```python
from build123d import *

# Parameters (mm, degrees)
ESQUISSE1_R             = 150
BOSS_EXTRU_1_DEPTH      = 2
ESQUISSE1_4_R           = 1.25
ENL_V_MAT_EXTRU_1_DEPTH = 1
ESQUISSE1_5_R           = 1.25
ENL_V_MAT_EXTRU_2_DEPTH = 13
BOSS_EXTRU_3_START      = 3
BOSS_EXTRU_3_DEPTH      = 3
BOSS_EXTRU_4_DEPTH      = 3
ENL_V_MAT_EXTRU_3_DEPTH = 50
CONG_1_R                = 1
ESQUISSE5_R             = 1
ENL_V_MAT_EXTRU_4_DEPTH = 180
ENL_V_MAT_EXTRU_5_DEPTH = 213.153246642
ESQUISSE7_W             = 7
ESQUISSE7_H             = 1
BOSS_EXTRU_5_DEPTH      = 20
CONG_3_R                = 1


with BuildPart() as part:
    # Esquisse1 → Boss.-Extru.1 (new body)
    with BuildSketch(Plane(origin=(0, 0, 0), x_dir=(1, 0, 0), z_dir=(0, 1, 0))):
        with Locations(Location((0, 0, 0), (0, 0, 270))):
            Circle(ESQUISSE1_R)
    extrude(amount=-BOSS_EXTRU_1_DEPTH)

    # Esquisse1<4> → Enlèv. mat.-Extru.1 (cut)
    with BuildSketch(Plane(origin=(0, 0, 0), x_dir=(1, 0, 0), z_dir=(0, 1, 0))):
        with BuildLine():
            Line((120, -88.323269867), (120, 88.323269867))
            ThreePointArc((120, 88.323269867), (-149, 0), (120, -88.323269867))
        make_face()
        with Locations(Location((0, -18.4, 0), (0, 0, 270))):
            Circle(ESQUISSE1_4_R, mode=Mode.SUBTRACT)
        with Locations(Location((0, -11, 0), (0, 0, 270))):
            Circle(ESQUISSE1_4_R, mode=Mode.SUBTRACT)
        Polygon((5, 7), (5, -6.999999465), (-5, -7), (-5.000000382, 7), align=None, mode=Mode.SUBTRACT)
        with Locations(Location((0, 11, 0), (0, 0, 270))):
            Circle(ESQUISSE1_4_R, mode=Mode.SUBTRACT)
        with Locations(Location((0, 18.4, 0), (0, 0, 270))):
            Circle(ESQUISSE1_4_R, mode=Mode.SUBTRACT)
    extrude(amount=-ENL_V_MAT_EXTRU_1_DEPTH, mode=Mode.SUBTRACT)

    # Esquisse1<5> → Enlèv. mat.-Extru.2 (cut)
    with BuildSketch(Plane(origin=(0, 0, 0), x_dir=(1, 0, 0), z_dir=(0, 1, 0))):
        Polygon((5, -6.999999465), (5, 7), (-5.000000382, 7), (-5, -7), align=None)
        with Locations(Location((0, -11, 0), (0, 0, 270))):
            Circle(ESQUISSE1_5_R)
        with Locations(Location((0, -18.4, 0), (0, 0, 270))):
            Circle(ESQUISSE1_5_R)
        with Locations(Location((0, 11, 0), (0, 0, 270))):
            Circle(ESQUISSE1_5_R)
        with Locations(Location((0, 18.4, 0), (0, 0, 270))):
            Circle(ESQUISSE1_5_R)
    extrude(amount=-ENL_V_MAT_EXTRU_2_DEPTH, mode=Mode.SUBTRACT)

    # Esquisse3 → Boss.-Extru.3 (add)
    with BuildSketch(Plane(origin=(0, 0, 0), x_dir=(1, 0, 0), z_dir=(0, 1, 0)).offset(BOSS_EXTRU_3_START)):
        with BuildLine():
            Line((120, -3.5), (149.959161107, -3.5))
            ThreePointArc((149.959161107, -3.5), (149.989789929, -1.750119126), (150, 0))
            ThreePointArc((150, 0), (149.989789929, 1.750119126), (149.959161107, 3.5))
            Line((149.959161107, 3.5), (120, 3.5))
            Line((120, 3.5), (120, -3.5))
        make_face()
    extrude(amount=-BOSS_EXTRU_3_DEPTH)

    # Esquisse3<2> → Boss.-Extru.4 (add)
    with BuildSketch(Plane(origin=(0, 0, 0), x_dir=(1, 0, 0), z_dir=(0, 1, 0))):
        with BuildLine():
            Line((120, -3.5), (149.959161107, -3.5))
            ThreePointArc((149.959161107, -3.5), (149.989789929, -1.750119126), (150, 0))
            ThreePointArc((150, 0), (149.989789929, 1.750119126), (149.959161107, 3.5))
            Line((149.959161107, 3.5), (120, 3.5))
            Line((120, 3.5), (120, -3.5))
        make_face()
    extrude(amount=-BOSS_EXTRU_4_DEPTH)

    # Esquisse4 → Enlèv. mat.-Extru.3 (cut)
    with BuildSketch(Plane(origin=(120, 0, 0), x_dir=(0, 0, -1), z_dir=(1, 0, 0))):
        with BuildLine():
            Line((-2, 1.5), (2, 1.5))
            ThreePointArc((2, 1.5), (2.5, 0), (2, -1.5))
            Line((2, -1.5), (-2, -1.5))
            ThreePointArc((-2, -1.5), (-2.5, 0), (-2, 1.5))
        make_face()
    extrude(amount=ENL_V_MAT_EXTRU_3_DEPTH, mode=Mode.SUBTRACT)

    # Congé1
    cong_1_edges = [part.edges().sort_by_distance(p)[0] for p in [
        (134.979580554, -3, -3.5),
        (134.979580554, -3, 3.5),
        (134.979580554, 3, 3.5),
        (134.979580554, 3, -3.5),
    ]]
    fillet(cong_1_edges, radius=CONG_1_R - 0.0001)  # a hair under: the kernel refuses the full size

    # Esquisse5 → Enlèv. mat.-Extru.4 (cut)
    with BuildSketch(Plane(origin=(0, 0, 0), x_dir=(0, 0, -1), z_dir=(1, 0, 0))):
        Circle(ESQUISSE5_R)
    extrude(amount=-ENL_V_MAT_EXTRU_4_DEPTH, mode=Mode.SUBTRACT)

    # Esquisse3<4> → Enlèv. mat.-Extru.5 (cut, through all)
    with BuildSketch(Plane(origin=(0, 0, 0), x_dir=(1, 0, 0), z_dir=(0, 1, 0))):
        with BuildLine():
            ThreePointArc((149.959161107, 3.5), (-150, 0), (149.959161107, -3.5))
            Line((149.959161107, -3.5), (120, -3.5))
            Line((120, -3.5), (120, -88.323269867))
            ThreePointArc((120, -88.323269867), (-149, 0), (120, 88.323269867))
            Line((120, 88.323269867), (120, 3.5))
            Line((120, 3.5), (149.959161107, 3.5))
        make_face()
    extrude(amount=-ENL_V_MAT_EXTRU_5_DEPTH, mode=Mode.SUBTRACT)

    # Esquisse7 → Boss.-Extru.5 (add)
    with BuildSketch(Plane.ZY.offset(-120)):
        with Locations((0, -2.5)):
            Rectangle(ESQUISSE7_W, ESQUISSE7_H)
    extrude(amount=BOSS_EXTRU_5_DEPTH)

    # Congé3
    cong_3_edges = [part.edges().sort_by_distance(p)[0] for p in [
        (100, -3, 0),
        (110, -3, -3.5),
        (110, -3, 3.5),
    ]]
    fillet(cong_3_edges, radius=CONG_3_R - 0.0001)  # a hair under: the kernel refuses the full size


solid = part.part
```
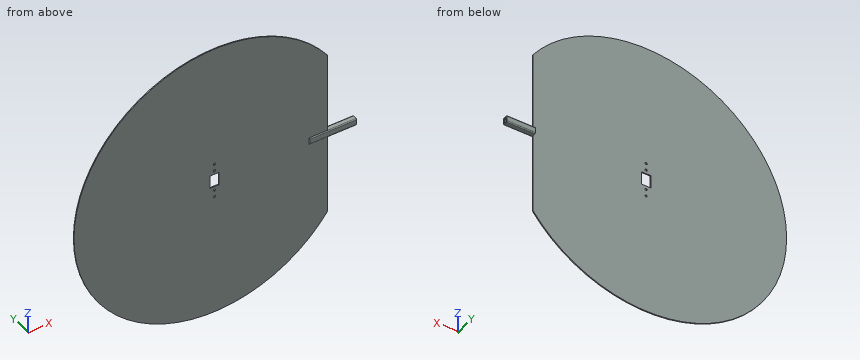
Geometry check sheet. Reference: the model listing, model coordinates, mm. Coordinates: 2 decimals unless noted, no trailing zeros. Order: outer loops, then holes, each group sorted by start corner. A loop starts at its lowest first (then second) coordinate and runs counter-clockwise, first axis right, second up. Notation, with made-up numbers: M 82,41 L 106,41 A25 cw 106,60 Z; hole C 25.5,26 d10. An arc over 180 degrees is marked long. Answer as a JSON object with one key per item and string values.
Q1. Cross-section at A-A on x = 90. Record the cut outline in (y, z).
Results are:
{"outline": "M -2,-118.75 L -1,-118.75 L -1,118.75 L -2,118.75 Z"}
Q2. Scan lines: line 1 (Y direction, x = 30, z = 2.5); line 2 (X direction, y = -1.65, z = -18.4); line 3 (X direction, y = -1.8, z = -11). Record each from-to range of solid material in increasing order.
Results are:
{"line 1": "y = -2 to -1", "line 2": "x = -147.86 to -1.25, 1.25 to 120", "line 3": "x = -148.59 to -1.25, 1.25 to 120"}
Q3. Depth check by flat-ended pin: pin 1 Ø0.5 at (y, z) = (-1.5, 40.5) entering from +X; pin 2 Ø3 at (x, z) = (0, 11) entering from -Y; pin 3 Ø0.5 at (y, z) = (-2.5, -3) entering from +X. Enter the tip coordinate at first touch or a pass-through.
Results are:
{"pin 1": "stops at x = 120", "pin 2": "stops at y = -2", "pin 3": "stops at x = 149.97"}
Q4. Cross-section at B-B on z = -36.5. Record the cut outline in (x, y), and give its area (3 significant figures).
Results are:
{"outline": "M -144.46,-2 L 120,-2 L 120,-1 L -144.46,-1 Z", "area": "264 mm²"}
